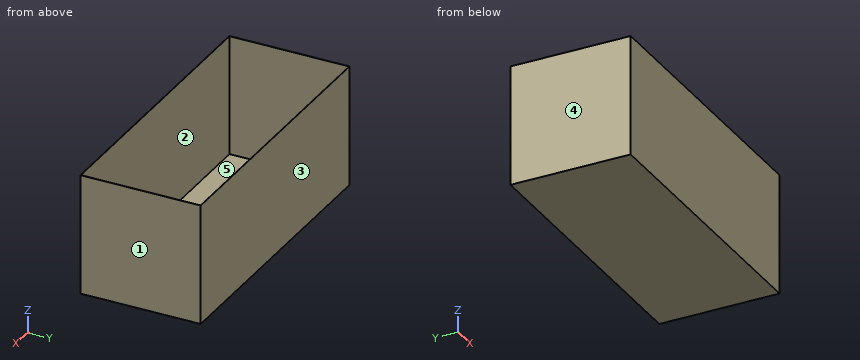
Solid Edge part; units mm, degrees
sketch "Sketch1" plane through (0, 0, 0) normal (0, 0, 1) x (1, 0, 0)
  line L0 (594, 249) -> (-594, 249)
  line L1 (-594, 249) -> (-594, -249)
  line L2 (-594, -249) -> (594, -249)
  line L3 (594, -249) -> (594, 249)
  line L4 (595, 250) -> (-595, 250)
  line L5 (-595, 250) -> (-595, -250)
  line L6 (-595, -250) -> (595, -250)
  line L7 (595, -250) -> (595, 250)
extrude "Protrusion1" add sketch "Sketch1" along normal blind 500
sketch "Sketch2" plane through (0, 0, 0) normal (0, 0, 1) x (1, 0, 0)
  line L0 (-594, -249) -> (594, -249)
  line L1 (594, -249) -> (594, 249)
  line L2 (594, 249) -> (-594, 249)
  line L3 (-594, 249) -> (-594, -249)
extrude "ExtrudedProtrusion_2" add sketch "Sketch2" along normal blind 2
properties material "Acrylic Plastic (extra strong)"
Input: part model. Units: mm. Frame: model coordinates. Face numbers are marked on the shaded views. A direction names the side the tool comes from. Coordinates: 2 decimals unless noted, no trailing zeros. Loops run counter-clockwise (first coordinate to the right, second up) from the corner with the lowest first, then second, coordinate; pieces in that order, holes last.
Q1. Contact query for flat-ended pins moving along their axis: pin 1 (6 mm diameter, centred on x = -320.5, y = -126.5, fed in from -Z); pin 2 (2 mm diameter, centred on x = 392, y = -80, fed in from +Z). Output: stop coordinate, or through.
Q2. Material intervals for line 1 (Y direction, x = -439.5, z = 393.5); line 2 (X direction, y = -146, z = 358); line 3 (Z direction, x = -189, y = -224), sorted ascending.
Q3. Draft query along Y for the marked faces 1, 2 and 3. Return one class per face: +Y half, -Y half, draft (parallel to the pull), parting line (faces both ways), or undercut.
Q4. Cut plane A-A (z = 298). Output: boundary loops of the cut face in (x, y).
Q5. Set-up query: the marked faces 4 and 5. Return all of +Z, -Z, +X, -X, +Y, -Y with unobstructed straight access to the full face (end or side cutting, diameter ignored); none if empty.
Q6. Cut plane B-B (x = -466). Output: boundary loops of the cut face in (y, z), then the cut area to 3 significant figures.
Q7. Cut plane C-C (y = 174.5). Output: boundary loops of the cut face in (x, z), then the cut area to 3 significant figures.
Working result:
1. pin 1: stops at z = 0
1. pin 2: stops at z = 2
2. line 1: y = -250 to -249, 249 to 250
2. line 2: x = -595 to -594, 594 to 595
2. line 3: z = 0 to 2
3. face 1: draft
3. face 2: undercut
3. face 3: +Y half
4. outline: (-595, -250) - (595, -250) - (595, 250) - (-595, 250) - close; hole (-594, -249) - (594, -249) - (594, 249) - (-594, 249) - close
5. face 4: +Z, -Z, -X, +Y, -Y
5. face 5: +Z
6. outline: (-250, 0) - (250, 0) - (250, 500) - (249, 500) - (249, 2) - (-249, 2) - (-249, 500) - (-250, 500) - close
6. area: 2,000 mm2
7. outline: (-595, 0) - (595, 0) - (595, 500) - (594, 500) - (594, 2) - (-594, 2) - (-594, 500) - (-595, 500) - close
7. area: 3,380 mm2
